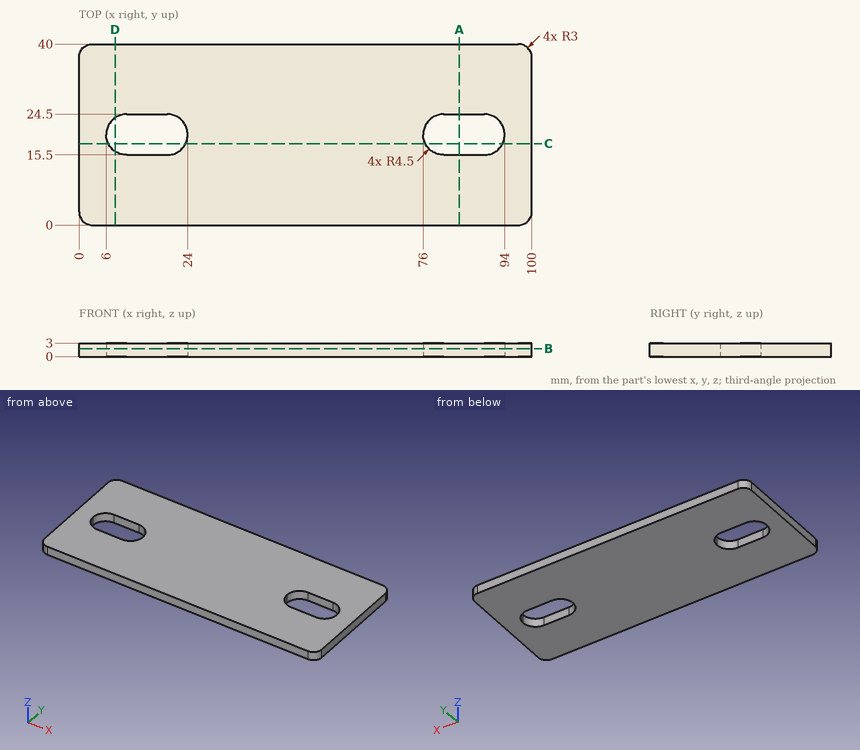
Geometry: see drawing. Coordinates: mm, zero at the bounding-box minimum. Coordinates: 2 decimals unless noted, no trailing zeros. Loops run counter-clockwise (first coordinate to the right, second up) from the corner with the lowest first, then second, coordinate; pieces in that order, holes last. Notation, with made-up numbers: (79, 43.5) -> (138, 43.5) arc R13 cw to (138, 50.5) -> close; hole circle Ø5 at (-1.5, -22.75). An arc over 180 degrees is marked (long way). Write item = value, one per line. Start each with the question number.
Item 1: Cut plane D-D, the plane x = 8. Return loops of the section in (y, z), plus the area to 4 significant figures.
Item 2: Cut plane C-C, the plane y = 18. Return loops of the section in (x, z).
Item 3: Cut plane A-A, the plane x = 84. Return loops of the section in (y, z).
Item 4: Material intervals for line 1 (X direction, y = 24, z = 1.7); line 2 (Y direction, x = 15, z = 1.5); line 3 (X direction, y = 21.5, z = 1.95), sorted ascending.
Item 5: Cut plane B-B, the plane z = 1.8. Count the separate pieces of the cut face and the enclosed holes in it, plus the area to 3 significant figures.
Ans:
q1.outline = (0, 0) -> (16.26, 0) -> (16.26, 3) -> (0, 3) -> close; (23.74, 0) -> (40, 0) -> (40, 3) -> (23.74, 3) -> close
q1.area = 97.55 mm²
q2.outline = (0, 0) -> (6.47, 0) -> (6.47, 3) -> (0, 3) -> close; (23.53, 0) -> (76.47, 0) -> (76.47, 3) -> (23.53, 3) -> close; (93.53, 0) -> (100, 0) -> (100, 3) -> (93.53, 3) -> close
q3.outline = (0, 0) -> (15.5, 0) -> (15.5, 3) -> (0, 3) -> close; (24.5, 0) -> (40, 0) -> (40, 3) -> (24.5, 3) -> close
q4.line_1 = 0 to 8.44, 21.56 to 78.44, 91.56 to 100
q4.line_2 = 0 to 15.5, 24.5 to 40
q4.line_3 = 0 to 6.26, 23.74 to 76.26, 93.74 to 100
q5.separate_pieces = 1
q5.enclosed_holes = 2
q5.area = 3,700 mm²
